The figure shows three views and two pictorial views of one solid part (mm, origin at its lowest corner). Answer the questions. Coordinates: 2 decimals unless noted, no trailing zeros. Loops run counter-clockwise (first coordinate to the right, second up) from the corner with the lowest first, then second, coordinate; pieces in that order, holes last. Notation, with made-up numbers: (32.5, 75) - (78.5, 75) arc R19 cw to (78.5, 98) - close; hole circle Ø2 at (48, 20). An arc over 180 degrees is marked (long way). Return JSON: item names as keys, results as strings. Group by question number.
1. Each of these flat-tipped pins is pushed along its axis until it touches: P1, Ø4.5, axis at x = 46, z = 7.5, coming from the +Y side; P2, Ø2, axis at x = 3.5, y = 2, coming from the -Z side; P3, Ø2, axis at y = 1, z = 18.5, coming from the +X side; P4, Ø1.3, axis at y = 1.5, z = 21.5, coming from the -X side. Where does it stop, or does it pass through?
2. Find the intervals of material crossed by line 1 along Z through (x, y) = (46, 1.2); line 2 along X through (y, z) = (3.75, 7.5); line 3 along Z through (x, y) = (34, 4.1), in increasing order.
3. Section C-C (z = 3.5) is taken. Write down the section's boundary in (x, y), and give its area (3 significant figures).
4. Section A-A (x = 46) is taken. Write down the section's boundary in (y, z), and give its area (3 significant figures).
5. Section B-B (y = 0.7) is taken. Write down the section's boundary in (x, z), and give its area (3 significant figures).
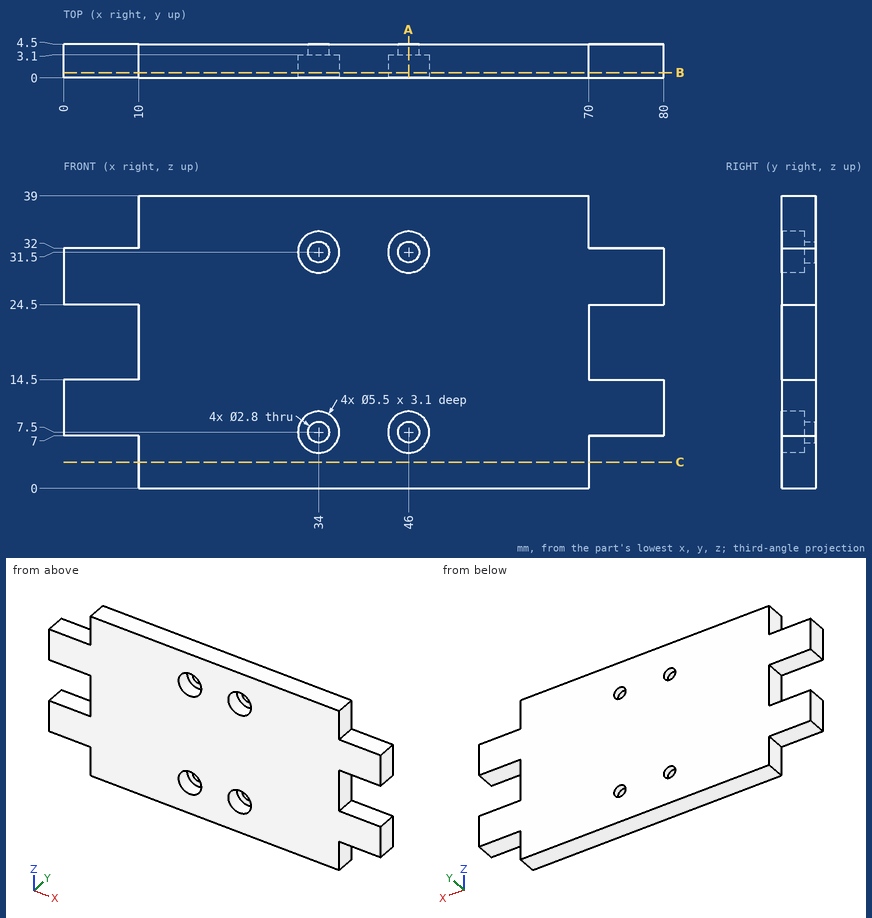
The answers:
{
 "1": {"P1": "stops at y = 4.5", "P2": "stops at z = 7", "P3": "stops at x = 70", "P4": "stops at x = 10"},
 "2": {"line 1": "z = 0 to 4.75, 10.25 to 28.75, 34.25 to 39", "line 2": "x = 0 to 32.6, 35.4 to 44.6, 47.4 to 80", "line 3": "z = 0 to 6.1, 8.9 to 30.1, 32.9 to 39"},
 "3": {"outline": "(10, 0) - (70, 0) - (70, 4.5) - (10, 4.5) - close", "area": "270 mm2"},
 "4": {"outline": "(0, 0) - (4.5, 0) - (4.5, 6.1) - (3.1, 6.1) - (3.1, 4.75) - (0, 4.75) - close; (0, 10.25) - (3.1, 10.25) - (3.1, 8.9) - (4.5, 8.9) - (4.5, 30.1) - (3.1, 30.1) - (3.1, 28.75) - (0, 28.75) - close; (0, 34.25) - (3.1, 34.25) - (3.1, 32.9) - (4.5, 32.9) - (4.5, 39) - (0, 39) - close", "area": "134 mm2"},
 "5": {"outline": "(0, 7) - (10, 7) - (10, 0) - (70, 0) - (70, 7) - (80, 7) - (80, 14.5) - (70, 14.5) - (70, 24.5) - (80, 24.5) - (80, 32) - (70, 32) - (70, 39) - (10, 39) - (10, 32) - (0, 32) - (0, 24.5) - (10, 24.5) - (10, 14.5) - (0, 14.5) - close; hole circle Ø5.5 at (34, 7.5); hole circle Ø5.5 at (34, 31.5); hole circle Ø5.5 at (46, 7.5); hole circle Ø5.5 at (46, 31.5)", "area": "2,540 mm2"}
}
